```python
from build123d import *

# Parameters (mm, degrees)
PAD011_DEPTH      = 1
SKETCH020_W       = 99
SKETCH020_H       = 70
PAD012_DEPTH      = 19
POCKET008_DEPTH   = 18
SKETCH023_R       = 4
SKETCH023_R_2     = 1.95
SKETCH023_R_3     = 2
PAD013_DEPTH      = 5.5
SKETCH024_R       = 1.95
POCKET010_DEPTH   = 8
PAD017_DEPTH      = 2.7
POCKET013_DEPTH   = 19
POCKET020_DEPTH   = 4
PAD033_START      = 34.8
PAD033_DEPTH      = 1
PAD034_START      = -34.8
PAD034_DEPTH      = 1
PAD035_START      = -35.8
SKETCH060_W       = 18
SKETCH060_H       = 18
PAD035_DEPTH      = 14
PAD036_START      = 35.8
PAD036_DEPTH      = 14
PAD037_DEPTH      = 15
PAD037_DEPTH_BACK = 15


with BuildPart() as part:
    # Sketch019 → Pad011 (new body)
    with BuildSketch(Plane.XY):
        with BuildLine():
            Line((-53.5, 45), (-53.5, -45))
            ThreePointArc((-53.5, -45), (-53.207107, -45.707107), (-52.5, -46))
            Line((-52.5, -46), (52.5, -46))
            ThreePointArc((52.5, -46), (53.207107, -45.707107), (53.5, -45))
            Line((53.5, -45), (53.5, 45))
            ThreePointArc((53.5, 45), (53.207107, 45.707107), (52.5, 46))
            Line((52.5, 46), (-52.5, 46))
            ThreePointArc((-52.5, 46), (-53.207107, 45.707107), (-53.5, 45))
        make_face()
    extrude(amount=PAD011_DEPTH)

    # Sketch020 → Pad012 (join)
    with BuildSketch(Plane.XY):
        with BuildLine():
            Line((-53.5, 45), (-53.5, -45))
            ThreePointArc((-53.5, -45), (-53.207107, -45.707107), (-52.5, -46))
            Line((-52.5, -46), (52.5, -46))
            ThreePointArc((52.5, -46), (53.207107, -45.707107), (53.5, -45))
            Line((53.5, -45), (53.5, 45))
            ThreePointArc((53.5, 45), (53.207107, 45.707107), (52.5, 46))
            Line((52.5, 46), (-52.5, 46))
            ThreePointArc((-52.5, 46), (-53.207107, 45.707107), (-53.5, 45))
        make_face()
        with Locations((0, -1)):
            Rectangle(SKETCH020_W, SKETCH020_H, mode=Mode.SUBTRACT)
    extrude(amount=PAD012_DEPTH)

    # Sketch021 (on Face14 of Pad012) → Pocket008 (cut)
    with BuildSketch(Plane.XY.offset(19)):
        with BuildLine():
            Line((-52.5, 45), (-52.5, 43.4))
            Line((-52.5, 43.4), (-10, 43.4))
            ThreePointArc((-8.5, 41.9), (-8.93934, 42.96066), (-10, 43.4))
            Line((-8.5, 41.9), (-8.5, 34))
            Line((-8.5, 34), (-7, 34))
            Line((-7, 34), (-7, 41.9))
            ThreePointArc((-5.5, 43.4), (-6.56066, 42.96066), (-7, 41.9))
            Line((-5.5, 43.4), (37, 43.4))
            Line((37, 43.4), (37, 37.5))
            Line((37, 37.5), (44, 37.5))
            Line((44, 37.5), (44, 34))
            Line((45.5, 34), (44, 34))
            Line((45.5, 37.5), (45.5, 34))
            Line((45.5, 37.5), (52.5, 37.5))
            Line((52.5, 45), (52.5, 37.5))
            Line((52.5, 45), (-52.5, 45))
        make_face()
    extrude(amount=-POCKET008_DEPTH, mode=Mode.SUBTRACT)

    # Sketch023 → Pad013 (join)
    with BuildSketch(Plane.XY):
        with Locations((31.5, 16)):
            Circle(SKETCH023_R)
        with Locations((31.5, 16)):
            Circle(SKETCH023_R_2, mode=Mode.SUBTRACT)
        with Locations((31.5, -6)):
            Circle(SKETCH023_R)
        with Locations((31.5, -6)):
            Circle(SKETCH023_R_2, mode=Mode.SUBTRACT)
        with Locations((0.5, 5)):
            Circle(SKETCH023_R_3)
    extrude(amount=PAD013_DEPTH)

    # Sketch024 (on Face14 of Pad013) → Pocket010 (cut)
    with BuildSketch(Plane.XY.offset(19)):
        with Locations((-48.5, -42)):
            Circle(SKETCH024_R)
        with Locations((-30, -42)):
            Circle(SKETCH024_R)
        with Locations((30, -42)):
            Circle(SKETCH024_R)
        with Locations((-48.5, 40)):
            Circle(SKETCH024_R)
        with Locations((-30, 40)):
            Circle(SKETCH024_R)
        with Locations((30, 40)):
            Circle(SKETCH024_R)
        with Locations((48.5, -42)):
            Circle(SKETCH024_R)
    extrude(amount=-POCKET010_DEPTH, mode=Mode.SUBTRACT)

    # Sketch025 (on Face4 of Pocket010) → Pad017 (join)
    with BuildSketch(Plane(origin=(0, 0, 0), x_dir=(1, 0, 0), z_dir=(0, 0, -1))):
        with BuildLine():
            Line((-50.500005, -36), (50.499995, -36))
            Line((50.499995, -36), (50.499995, 46))
            Line((52.5, 46), (50.499995, 46))
            ThreePointArc((53.5, 45), (53.207107, 45.707107), (52.5, 46))
            Line((53.5, -36), (53.5, 45))
            ThreePointArc((52.5, -37), (53.207107, -36.707107), (53.5, -36))
            Line((-52.5, -37), (52.5, -37))
            ThreePointArc((-53.5, -36), (-53.207107, -36.707107), (-52.5, -37))
            Line((-53.5, 45), (-53.5, -36))
            ThreePointArc((-52.500009, 46), (-53.20711, 45.707104), (-53.5, 45))
            Line((-52.500009, 46), (-50.500005, 46))
            Line((-50.500005, 46), (-50.500005, -36))
        make_face()
    extrude(amount=PAD017_DEPTH)

    # Sketch026 → Pocket013 (cut)
    with BuildSketch(Plane.XY):
        with BuildLine():
            ThreePointArc((-10, 0.5), (-15, -4.5), (-10, -9.5))
            Line((-10, -9.5), (10, -9.5))
            ThreePointArc((10, -9.5), (15, -4.5), (10, 0.5))
            Line((-10, 0.5), (10, 0.5))
        make_face()
    extrude(amount=POCKET013_DEPTH, mode=Mode.SUBTRACT)

    # Sketch053 (on Face18 of Pocket013) → Pocket020 (cut)
    with BuildSketch(Plane.XY.offset(19)):
        Polygon((-52.5, 43.4), (-52.5, -39), (52.5, -39), (52.5, 37.5), (50.9, 37.5), (50.9, 34), (47.9, 34), (47.9, 32.4), (50.9, 32.4), (50.9, -37.4), (-50.9, -37.4), (-50.9, 32.4), (-47.9, 32.4), (-47.9, 34), (-50.9, 34), (-50.9, 43.4), align=None)
    extrude(amount=-POCKET020_DEPTH, mode=Mode.SUBTRACT)

    # Sketch059 → Pad033 (join)
    with BuildSketch(Plane.YZ.offset(PAD033_START)):
        Polygon((-36, 19), (-36, 1), (-18, 1), (-18, 4), (-32, 4), (-32, 19), align=None)
    extrude(amount=PAD033_DEPTH)

    # Sketch059 → Pad034 (join)
    with BuildSketch(Plane.YZ.offset(PAD034_START)):
        Polygon((-36, 19), (-36, 1), (-18, 1), (-18, 4), (-32, 4), (-32, 19), align=None)
    extrude(amount=-PAD034_DEPTH)

    # Sketch060 → Pad035 (join)
    with BuildSketch(Plane.YZ.offset(PAD035_START)):
        with Locations((-27, 10)):
            Rectangle(SKETCH060_W, SKETCH060_H)
    extrude(amount=-PAD035_DEPTH)

    # Sketch060 → Pad036 (join)
    with BuildSketch(Plane.YZ.offset(PAD036_START)):
        with Locations((-27, 10)):
            Rectangle(SKETCH060_W, SKETCH060_H)
    extrude(amount=PAD036_DEPTH)

    # Sketch056 → Pad037 (join, two sides)
    with BuildSketch(Plane.YZ) as pad037_sk:
        with BuildLine():
            add(Edge.make_bspline(
                [(-21, 17), (-18, 17), (-18, 10.5)],
                knots=[0, 0, 0, 1, 1, 1], degree=2, weights=[1, 0.5, 1]))
            Line((-18, 10.5), (-18, 1))
            Line((-18, 1), (-15, 1))
            Line((-15, 1), (-18, 17))
            Line((-18, 17), (-21, 17))
        make_face()
    extrude(amount=PAD037_DEPTH)
    extrude(pad037_sk.sketch, amount=-PAD037_DEPTH_BACK)


solid = part.part
```
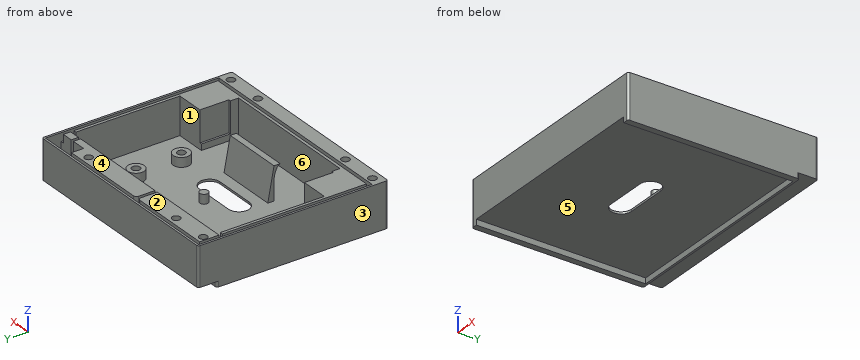
For this review, take the finished solid that the model builds, in its own axes (mm). Face numbers are marked on the shaded views. A direction names the side the tool comes from. Round coordinates to 2 decimals unless told otherwise and drop trailing zeros. Write each loop counter-clockwise with the first axis right and the second up, starting at its lowest first coordinate (ties: lowest second). Pieces come first, ordered by that corner, then holes. Notation, with made-up numbers: (46.5, 34) - (56.5, 34) arc R22 ccw to (56.5, 72) - close; hole circle Ø9 at (20.25, 45.5). An arc over 180 degrees is marked (long way). Put each result on its own line as item: value.
Q1. We need section A-A (y = 5). Give the boundary of the cut face in (x, z), and give its area (3 significant figures).
Solved:
outline: (-53.5, -2.7) - (-50.5, -2.7) - (-50.5, 0) - (50.5, 0) - (50.5, -2.7) - (53.5, -2.7) - (53.5, 19) - (52.5, 19) - (52.5, 15) - (50.9, 15) - (50.9, 19) - (49.5, 19) - (49.5, 1) - (2.5, 1) - (2.5, 5.5) - (-1.5, 5.5) - (-1.5, 1) - (-49.5, 1) - (-49.5, 19) - (-50.9, 19) - (-50.9, 15) - (-52.5, 15) - (-52.5, 19) - (-53.5, 19) - close
area: 272 mm2
Q2. Wall thickness on probe 1 along Y at (x, z) = (21.5, 9); probe 2 along Y at (x, z) = (-48.5, 13); probe 3 along Y at (x, z) = (48.5, 16): over which ranges is each line inside the solid? List them lowest first.
Solved:
probe 1: y = -46 to -36, 34 to 43.4, 45 to 46
probe 2: y = -46 to -43.95, -40.05 to -18, 34 to 38.05, 41.95 to 43.4, 45 to 46
probe 3: y = -46 to -43.95, -40.05 to -39, -37.4 to -18, 34 to 37.5, 45 to 46
Q3. Mouldability with a two-part tool opening along X and no side actions: class the marked faces 1, 2 and 3 as released by +X, released by -X, zero draft, split by the parting line, or undercut.
Solved:
face 1: undercut
face 2: zero draft
face 3: released by -X
Q4. We need section C-C (y = 16). Give the boundary of the cut face in (x, z).
Solved:
outline: (-53.5, -2.7) - (-50.5, -2.7) - (-50.5, 0) - (50.5, 0) - (50.5, -2.7) - (53.5, -2.7) - (53.5, 19) - (52.5, 19) - (52.5, 15) - (50.9, 15) - (50.9, 19) - (49.5, 19) - (49.5, 1) - (35.5, 1) - (35.5, 5.5) - (33.45, 5.5) - (33.45, 1) - (29.55, 1) - (29.55, 5.5) - (27.5, 5.5) - (27.5, 1) - (-49.5, 1) - (-49.5, 19) - (-50.9, 19) - (-50.9, 15) - (-52.5, 15) - (-52.5, 19) - (-53.5, 19) - close
Q5. We need section D-D (y = -27). Give the boundary of the cut face in (x, z), and give its area (3 significant figures).
Solved:
outline: (-53.5, -2.7) - (-50.5, -2.7) - (-50.5, 0) - (50.5, 0) - (50.5, -2.7) - (53.5, -2.7) - (53.5, 19) - (52.5, 19) - (52.5, 15) - (50.9, 15) - (50.9, 19) - (35.8, 19) - (35.8, 4) - (34.8, 4) - (34.8, 1) - (-34.8, 1) - (-34.8, 4) - (-35.8, 4) - (-35.8, 19) - (-50.9, 19) - (-50.9, 15) - (-52.5, 15) - (-52.5, 19) - (-53.5, 19) - close
area: 754 mm2
Q6. Insertion check: pin 1 Ø1 at (x, y) = (42.5, 21.5) entering from +Z; pin 2 Ø3 at (x, y) = (48.5, -42) entering from +Z; pin 3 Ø3 at (x, y) = (31.5, -6.5) entering from +Z. Each pin has a flat end and moves straight along its axis. Give the tip position at first contact, or say it passes through.
Solved:
pin 1: stops at z = 1
pin 2: stops at z = 11
pin 3: stops at z = 5.5
Q7. We need section B-B (z = 7). Count the separate pieces of the cut face and the enclosed holes in it, and give its area (3 significant figures).
Solved:
separate pieces: 3
enclosed holes: 1
area: 3,190 mm2
Q8. Machinability: for the marked faces 4, 5 and 6, which of the approach directions +Z, -Z, +X, -X, +Y, -Y give a long, thin tool a straight path to every point of the face, cutting with its end or side? Answer none if there is none.
Solved:
face 4: +Z, +X, -X, +Y, -Y
face 5: -Z, -Y
face 6: +Z
